CAD build for the part. Positions are in the model's coordinates, mm. A direction names the side the tool comes from. Give positions to 0.01 mm unless a question says otherwise; leave off trailing zeros. Answer as CSV lines item,"result".
Autodesk Inventor part; units mm, degrees
ref_plane "Work Plane3" through (60, 34, 18) normal (1, 0, 0) x (0, 1, 0)
ref_plane "XZ Plane" through (0, 0, 0) normal (0, 1, 0) x (-1, 0, 0)
ref_plane "XY Plane" through (0, 0, 0) normal (0, 0, 1) x (1, 0, 0)
sketch "Sketch1" plane through (0, 0, 0) normal (0, 0, 1) x (1, 0, 0)
  line L0 (60, 34) -> (279, 34) construction
  line L1 (279, 34) -> (279, 16) construction
  line L2 (279, 16) -> (60, 16) construction
  line L3 (60, 16) -> (60, 34) construction
  line L4 (158.3401, 144) -> (180.6599, 144)
  line L5 (-98.1271, 119.3914) -> (-155.2055, 119.3914) construction
  line L6 (60, 204.7828) -> (279, 204.7828) construction
  line L7 (279, 204.7828) -> (279, 222.7828) construction
  line L8 (279, 222.7828) -> (60, 222.7828) construction
  line L9 (60, 222.7828) -> (60, 204.7828) construction
  line L10 (158.3401, 94.7828) -> (180.6599, 94.7828) construction
  line L11 (169.5, 144) -> (169.5, 94.7828) construction
  circle A0 centre (169.5, 144.5) radius 4.5 construction
  circle A1 centre (169.5, 94.2828) radius 4.5 construction
  line L12 (165, 140) -> (174, 140) construction
  spline S0 degree 4 poles (60, 34) (60, 50.8003) (67.6192, 82.543) (79.1211, 110.1157) (114.0169, 138.9549) (142.0747, 144) (158.3401, 144) knots 0 0 0 0 0 0.37584 0.62584 1 1 1 1 1
  line L13 (436.9307, -63.7999) -> (436.9307, -111.3151) construction
  line L14 (165.0658, 130) -> (173.4412, 130)
  line L15 (173.4412, 130) -> (178.3964, 144)
  line L16 (178.3964, 144) -> (180.6599, 144)
  line L17 (166.2744, 149) -> (172.7256, 149) construction
  spline S1 degree 4 poles (165.0658, 130) (150.6222, 130) (124.5762, 123.7444) (97.0964, 105.142) (83.3994, 60.1633) (114.2343, 37) (132, 37) knots 0 0 0 0 0 0.366098 0.616098 1 1 1 1 1
  line L18 (158.3401, 94.7828) -> (180.6599, 94.7828) construction
  line L19 (178.3964, 94.7828) -> (180.6599, 94.7828) construction
  line L20 (180.6599, 94.7828) -> (158.3401, 94.7828) construction
  spline S2 degree 4 poles (173.9342, 106.4847) (188.3699, 106.4847) (225.2165, 124.0597) (250.4536, 142.2568) (239.0722, 211.617) (207.7908, 202.4847) knots 0 0 0 0 0 0.376784 1 1 1 1 1 construction
  spline S3 degree 4 poles (279, 204.7828) (275.6992, 148.3745) (255.9313, 132.0927) (229.7092, 97.2581) (180.6599, 94.7828) knots 0 0 0 0 0 1 1 1 1 1 construction
  line L21 (173.9342, 106.4847) -> (158.8804, 106.4847) construction
  line L22 (160.6036, 94.7828) -> (158.3401, 94.7828) construction
  line L23 (158.8804, 106.4847) -> (160.6036, 94.7828) construction
  arc A2 (135, 34) -> (132, 37) centre (132, 34) ccw
  line L24 (135, 34) -> (60, 34)
  point P0 (0, 0)
  point P1 (169.5, 34)
  point P2 (169.5, 204.7828)
  point P3 (93.4315, 204.7828)
  point P4 (169.5, 140)
  point P5 (69.0653, 81.3021)
  point P6 (84.771, 109.712)
  point P7 (114.2865, 133.8506)
  point P8 (169.5, 149)
  point P9 (126.5497, 121.1282)
  point P10 (101.7633, 99.5435)
  point P11 (94.9383, 64.5723)
  point P12 (209.9254, 118.4197)
  point P13 (233.3153, 142.9189)
  point P14 (236.6483, 184.5924)
  point P15 (268.3461, 156.1626)
  point P16 (250.8428, 129.4297)
  point P17 (224.4145, 107.9607)
  dimension "d0" = 18
  dimension "d2" = 219
  dimension "d4" = 16
  dimension "d5" = 60
  dimension "d6" = 110
  dimension "d9" = 9
  dimension "d11" = 10
  dimension "exposed" = 5
  dimension "d13" = 14
  dimension "d23" = 3
  dimension "d43" = 75
  dimension "d48" = 109.5
extrude "Extrusion1" add sketch "Sketch1" along normal blind 18
sketch "Sketch4" plane through (158.3401, 144, 0) normal (0, 1, 0) x (1, 0, 0)
  line L0 (-98.3401, -118.5) -> (120.6599, -118.5) construction
  line L1 (120.6599, -118.5) -> (120.6599, 100.5) construction
  line L2 (120.6599, 100.5) -> (-98.3401, 100.5) construction
  circle A0 centre (11.1599, -9) radius 1
  line L3 (-98.3401, 0) -> (-98.3401, -18)
  line L4 (20.0563, 0) -> (20.0563, -18)
  point P0 (-158.3401, 0)
  point P1 (11.1599, -118.5)
  point P2 (120.6599, -9)
  point P3 (20.0563, -9)
  dimension "d30" = 219
  dimension "d31" = 219
  dimension "d32" = 2
  dimension "d49" = 109.5
extrude "Extrusion5" cut sketch "Sketch4" against normal through all
sketch "Sketch5" plane through (158.3401, 144, 0) normal (0, 1, 0) x (1, 0, 0)
  line L0 (26.7348, -7.5) -> (5.6599, -7.5)
  line L1 (5.6599, -7.5) -> (5.6599, -10.5)
  line L2 (5.6599, -10.5) -> (26.7348, -10.5)
  line L3 (26.7348, -10.5) -> (26.7348, -7.5)
  circle A0 centre (11.1599, -9) radius 1
  line L4 (6.6599, -8.6) -> (15.6599, -8.6) construction
  line L5 (15.6599, -8.6) -> (15.6599, -9.4) construction
  line L6 (15.6599, -9.4) -> (6.6599, -9.4) construction
  line L7 (6.6599, -9.4) -> (6.6599, -8.6) construction
  point P0 (-158.3401, 0)
  point P1 (5.6599, -9)
  point P2 (6.6599, -9)
  point P3 (11.1599, -8.6)
  point P4 (11.1599, -10.5)
  point P5 (11.1599, -7.5)
  dimension "d35" = 3
  dimension "d36" = 9
  dimension "d37" = 0.8
  dimension "d41" = 1
extrude "Extrusion6" cut sketch "Sketch5" against normal blind 4 contours L3 L2 L1 L0 | A0
ref_plane "Work Plane3" through (60, 34, 18) normal (1, 0, 0) x (0, 1, 0)
sketch "Sketch6" plane through (60, 34, 18) normal (1, 0, 0) x (0, 1, 0)
  line L0 (-13, -18) -> (-13, 0)
  line L1 (0, -18) -> (0, 0)
  line L2 (-13, -18) -> (0, -15.8012)
  line L3 (0, -18) -> (0, 0)
  line L4 (0, -15.8012) -> (-9.0304, -15.8012) construction
  line L5 (-15.1424, -9) -> (-18.4796, -9) construction
  line L6 (-13, 0) -> (0, -2.1988)
  point P0 (-34, -18)
  point P1 (-16.811, -9)
  point P2 (-13, -9)
  dimension "d44" = 13
  dimension "d45" = 9.6
extrude "Extrusion7" add sketch "Sketch6" along normal up to surface (75 mm away)
properties part number "TNS-1-arm"
Q1. Wall check: line 1 (Z direction, x = 169.5, y = 137.75); line 2 (X direction, y = 134.75, z = 9); line 3 (X direction, y = 31.5, z = 3.5). Give the ranges that are in metal, low to high. Write a range as [from, to].
Solution:
line 1,"z = [0, 8], [10, 18]"
line 2,"x = [116.08, 168.5], [170.5, 175.12]"
line 3,"x = [60, 135]"
Q2. Pin check, flat tips, straight feed: P1, Ø2.5, axis at x = 169.5, z = 9, coming from the +Y side; P2, Ø6, axis at y = 67, z = 7.5, coming from the +X side; P3, Ø3, axis at y = 55, z = 4.5, coming from the +X side; P4, Ø1.2, axis at x = 169, y = 142, coming from the -Z side. Stop position of each tip, or through.
Solution:
P1,"stops at y = 140"
P2,"stops at x = 95.12"
P3,"stops at x = 100.63"
P4,"stops at z = 0"
Q3. Which spindle directions (+Z, -Z, +X, -X, +Y, -Y) get a long thin tool onto all of the face, cutting with end or side? Do faces 1 (the flat face through (96.975, 27.409, 16.916)), 2 (the flat face through (170.4, 140, 10)), 3 (the flat face through (168, 130, 9)). Say none if no direction does.
Solution:
face 1,"+Z, +X, -X"
face 2,"+X, +Y"
face 3,"+Z, -Z, +X, -Y"
Q4. Mould opens along Z. For faces 4 (the flat face through (96.975, 27.409, 1.084)), 5 (the flat face through (164, 142, 9)), 6 (the flat face through (171, 142, 10.5)), 7 (the cylindrical face through (134.1, 36.14, 8.87)) say: released by +Z, released by -Z, zero draft, split by the parting line, or undercut.
Solution:
face 4,"released by -Z"
face 5,"undercut"
face 6,"undercut"
face 7,"zero draft"
